Drawing for the job (mm, zero at the part's lowest x, y, z). Round coordinates to 2 decimals unless told otherwise and drop trailing zeros. Write each loop counter-clockwise with the first axis right and the second up, starting at its lowest first coordinate (ties: lowest second). Pieces come first, ordered by that corner, then holes.
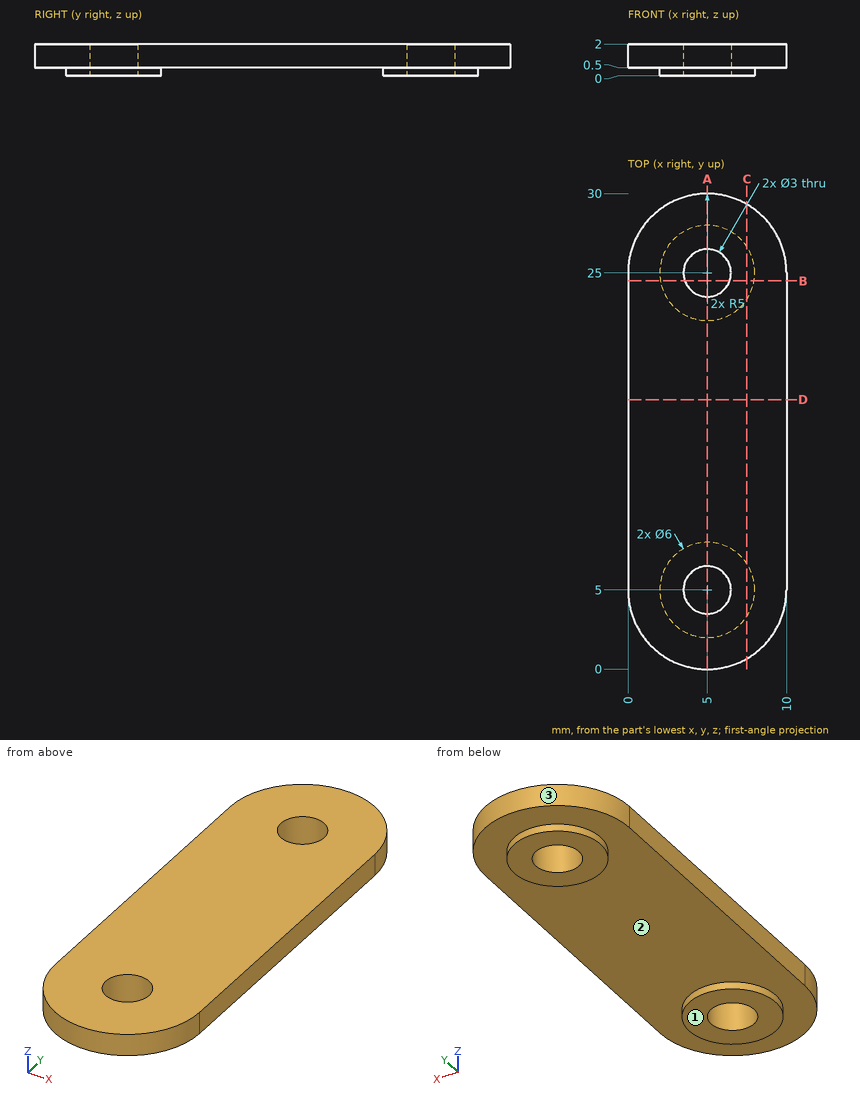
Q1. Saw through at A-A, the plane x = 5. Write the cut outline in (y, z), and give its area (3 significant figures).
Q2. Two-plate mould, pull along Y, no slides. Class the marked faces 1, 2 and 3: released by +Y, released by -Y, zero draft, split by the parting line, or undercut.
Q3. Saw through at C-C, the plane x = 7.5. Write the cut outline in (y, z), and give its area (3 significant figures).
Q4. Saw through at B-B, the plane y = 24.5. Write the cut outline in (x, z), and give its area (3 significant figures).
Q5. Wall check: line 1 (Y direction, x = 5, z = 0.9); line 2 (Y direction, x = 6, z = 0.35); line 3 (Z direction, x = 8.75, y = 27.5). Give the ranges that are in metal, low to high.
Q6. Saw through at D-D, the plane y = 17. Write the cut outline in (x, z), and give its area (3 significant figures).
Q7. Drop flat-ended pins along their axis: P1, Ø2.5, axis at x = 5, y = 5, coming from the -Z side; P2, Ø4, axis at x = 6.5, y = 11.5, coming from the -Z side; P3, Ø1, axis at x = 1.5, z = 1, coming from the +Y side. Give the stop position or say it passes through.
Computed:
1. outline: (0, 0.5) - (2, 0.5) - (2, 0) - (3.5, 0) - (3.5, 2) - (0, 2) - close; (6.5, 0) - (8, 0) - (8, 0.5) - (22, 0.5) - (22, 0) - (23.5, 0) - (23.5, 2) - (6.5, 2) - close; (26.5, 0) - (28, 0) - (28, 0.5) - (30, 0.5) - (30, 2) - (26.5, 2) - close
1. area: 39.0 mm2
2. face 1: zero draft
2. face 2: undercut
2. face 3: released by +Y
3. outline: (0.67, 0.5) - (3.34, 0.5) - (3.34, 0) - (6.66, 0) - (6.66, 0.5) - (23.34, 0.5) - (23.34, 0) - (26.66, 0) - (26.66, 0.5) - (29.33, 0.5) - (29.33, 2) - (0.67, 2) - close
3. area: 46.3 mm2
4. outline: (0, 0.5) - (2.04, 0.5) - (2.04, 0) - (3.59, 0) - (3.59, 2) - (0, 2) - close; (6.41, 0) - (7.96, 0) - (7.96, 0.5) - (10, 0.5) - (10, 2) - (6.41, 2) - close
4. area: 12.3 mm2
5. line 1: y = 0 to 3.5, 6.5 to 23.5, 26.5 to 30
5. line 2: y = 2.17 to 3.88, 6.12 to 7.83, 22.17 to 23.88, 26.12 to 27.83
5. line 3: z = 0.5 to 2
6. outline: (0, 0.5) - (10, 0.5) - (10, 2) - (0, 2) - close
6. area: 15.0 mm2
7. P1: passes through
7. P2: stops at z = 0.5
7. P3: stops at y = 29
